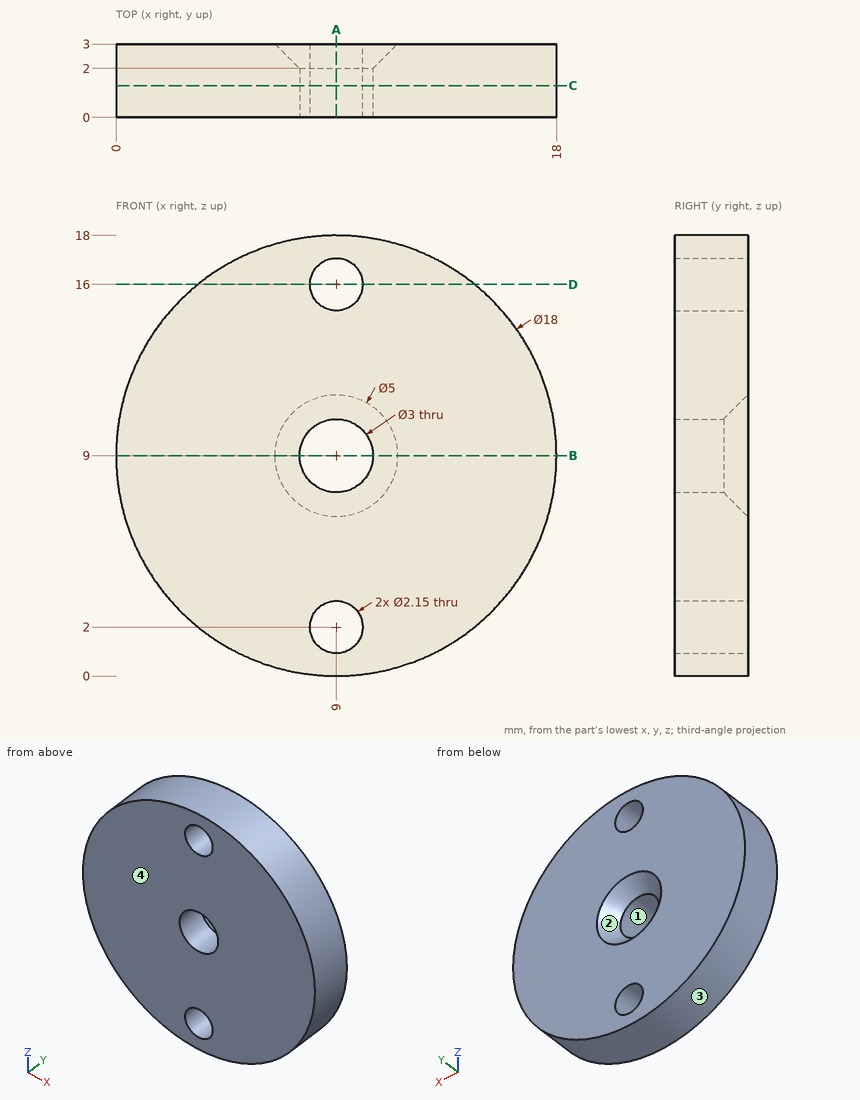
Design review of the part shown in the three views and the two pictorial views. Dimensions are in mm from the part's minimum x, y and z. Coordinates: 2 decimals unless noted, no trailing zeros. Loops run counter-clockwise (first coordinate to the right, second up) from the corner with the lowest first, then second, coordinate; pieces in that order, holes last.
Q1. We need section B-B on z = 9. State the section outline as (x, y) points, and give its area (3 significant figures).
Reported:
outline: (0, 0) - (7.5, 0) - (7.5, 2) - (6.5, 3) - (0, 3) - close; (10.5, 0) - (18, 0) - (18, 3) - (11.5, 3) - (10.5, 2) - close
area: 44.0 mm2
Q2. We need section D-D on z = 16. State the section outline as (x, y) points (3 decimals).
Reported:
outline: (3.343, 0) - (7.925, 0) - (7.925, 3) - (3.343, 3) - close; (10.075, 0) - (14.657, 0) - (14.657, 3) - (10.075, 3) - close
Q3. To check wall thickness, follow line 1 (Z direction, x = 9, y = 1.65) (3 decimals); line 2 (Z direction, x = 9, y = 2.35) (3 decimals); line 3 (X direction, y = 2.6, z = 7.5). State the ranges of each line that lie inside material, in increasing order.
Reported:
line 1: z = 0 to 0.925, 3.075 to 7.5, 10.5 to 14.925, 17.075 to 18
line 2: z = 0 to 0.925, 3.075 to 7.15, 10.85 to 14.925, 17.075 to 18
line 3: x = 0.13 to 7.53, 10.47 to 17.87
Q4. We need section A-A on x = 9. State the section outline as (y, z) points (3 decimals).
Reported:
outline: (0, 0) - (3, 0) - (3, 0.925) - (0, 0.925) - close; (0, 3.075) - (3, 3.075) - (3, 6.5) - (2, 7.5) - (0, 7.5) - close; (0, 10.5) - (2, 10.5) - (3, 11.5) - (3, 14.925) - (0, 14.925) - close; (0, 17.075) - (3, 17.075) - (3, 18) - (0, 18) - close
Q5. The part is to be moulded in two halves that separate along X. For the marked faces 1, 2, 3 and 4, say which applies: +X half, -X half, draft (parallel to the pull), parting line (faces both ways), or undercut.
Reported:
face 1: undercut
face 2: undercut
face 3: parting line
face 4: draft
Q6. We need section C-C on y = 1.3. State the section outline as (x, z) points (3 decimals).
Reported:
outline: circle Ø18 at (9, 9); hole circle Ø3 at (9, 9); hole circle Ø2.15 at (9, 2); hole circle Ø2.15 at (9, 16)
